Design review of the part built by this model. Coordinates are the model's own, in mm. A direction names the side the tool comes from. Give positions to 0.01 mm unless a question says otherwise; leave off trailing zeros. Write each loop counter-clockwise with the first axis right and the second up, starting at its lowest first coordinate (ties: lowest second). Pieces come first, ordered by that corner, then holes. Notation, with made-up numbers: M 14,66.5 L 23,66.5 A31 ccw 23,93.5 Z; hole C 66.25,74 d9. An arc over 180 degrees is marked long. Answer in a Markdown table with one row per item.
```python
from build123d import *

# Parameters (mm, degrees)
F0_W     = 140
F0_H     = 320
F1_DEPTH = 4.826
F2_W     = 31.75
F2_H     = 31.75
F2_W_2   = 25.4
F2_H_2   = 25.4
F3_DEPTH = 320
F4_W     = 25.4
F4_H     = 25.4
F4_W_2   = 15.874
F4_H_2   = 15.874
F5_DEPTH = 25
F6_R     = 2
F7_DEPTH = 4
F8_R     = 2.5
F8_R_2   = 3
F9_DEPTH = 4


with BuildPart() as f1:
    # F0 (on Top) → F1 (new body)
    with BuildSketch(Plane.XY):
        with Locations((-1.276044, 117.026612)):
            Rectangle(F0_W, F0_H)
    extrude(amount=F1_DEPTH)

    # F2 (on face) → F3 (join)
    with BuildSketch(Plane.XZ.offset(42.973388)):
        with Locations((-55.401044, -15.875)):
            Rectangle(F2_W, F2_H)
        with Locations((-55.401044, -15.875)):
            Rectangle(F2_W_2, F2_H_2, mode=Mode.SUBTRACT)
        with Locations((52.848956, -15.875)):
            Rectangle(F2_W, F2_H)
        with Locations((52.848956, -15.875)):
            Rectangle(F2_W_2, F2_H_2, mode=Mode.SUBTRACT)
    extrude(amount=-F3_DEPTH)

    # F4 (on face) → F5 (join, symmetric)
    with BuildSketch(Plane.XZ.offset(42.973388)):
        with Locations((-55.401044, -15.875)):
            Rectangle(F4_W, F4_H)
        with Locations((-55.401044, -15.875)):
            Rectangle(F4_W_2, F4_H_2, mode=Mode.SUBTRACT)
        with Locations((52.848956, -15.875)):
            Rectangle(F4_W, F4_H)
        with Locations((52.848956, -15.875)):
            Rectangle(F4_W_2, F4_H_2, mode=Mode.SUBTRACT)
    extrude(amount=F5_DEPTH, both=True)

    # F6 (on face) → F7 (cut)
    with BuildSketch(Plane.YZ.offset(-39.526044)):
        with Locations((117.026612, -21.75)):
            Circle(F6_R)
    extrude(amount=-F7_DEPTH, mode=Mode.SUBTRACT)

    # F8 (on face) → F9 (cut)
    with BuildSketch(Plane.XY.offset(4.826)):
        with Locations((-36.276044, -22.973388)):
            Circle(F8_R)
        with Locations((28.723956, -32.973388)):
            Circle(F8_R_2)
    extrude(amount=-F9_DEPTH, mode=Mode.SUBTRACT)


solid = f1.part
```
1) The part is to be moulded in two halves that separate along Z. For faces 6 (the face through (-42.701, 127, -16)), 7 (the face through (40.149, -56, -16)), 8 (the face through (-56, -55, -3.175)), say which applies: released by +Z, released by -Z, zero draft, split by the parting line, or undercut.
Geometry says:
| item | result |
|---|---|
| face 6 | undercut |
| face 7 | zero draft |
| face 8 | released by +Z |
2) Add section A-A (y = 71). Write out the cut boundary in (x, z) (3 decimals).
Geometry says:
| item | result |
|---|---|
| outline | M -71.276,-31.75 L -39.526,-31.75 L -39.526,0 L 36.974,0 L 36.974,-31.75 L 68.724,-31.75 L 68.724,4.826 L -71.276,4.826 Z; hole M -68.101,-28.575 L -42.701,-28.575 L -42.701,-3.175 L -68.101,-3.175 Z; hole M 40.149,-28.575 L 65.549,-28.575 L 65.549,-3.175 L 40.149,-3.175 Z |
3) To check wall thickness, follow probe 1 along X at (y, z) = (146, -15.5); probe 2 along Z at (x, y) = (-65.5, 92) (3 decimals); probe 3 along Z at (x, y) = (-39, 94.5). State the ranges of each line that lie inside material, in increasing order. Write a range as [from, to].
Geometry says:
| item | result |
|---|---|
| probe 1 | [-71.28, -68.1], [-42.7, -39.53], [36.97, 40.15], [65.55, 68.72] |
| probe 2 | [-31.75, -28.575], [-3.175, 4.826] |
| probe 3 | [0, 4.83] |
4) Add section B-B (x = -21). Write out the cut boundary in (y, z).
Geometry says:
| item | result |
|---|---|
| outline | M -42.97,0 L 277.03,0 L 277.03,4.83 L -42.97,4.83 Z |
5) Insertion check: P1, Ø5, axis at x = -33, y = 81, coming from the -Z side; P2, Ø8, axis at x = -58.5, y = -51.5, coming from the +Z side (3 decimals); P3, Ø5, axis at x = -57.5, y = -46, coming from the -Z side (3 decimals). Each pin has a flat end and moves straight along its axis. Give the tip position at first contact, or say it passes through.
Geometry says:
| item | result |
|---|---|
| P1 | z = 0 |
| P2 | z = -3.175 |
| P3 | z = -28.575 |
6) For faces 1 (the face through (36.974, 115, -16)), 2 (the face through (-56, 127, -3.175)), 3 (the face through (53, -56, -3.175)), 4 (the face through (-42.701, -55, -16)), 5 (the face through (60.786, -43, -16)), list the 3-axis set-ups (+Z, -Z, +X, -X, +Y, -Y) from which the entire face can be reached by the end or side of a thin tool; tool diameter is ignored.
Geometry says:
| item | result |
|---|---|
| face 1 | -Z, +Y, -Y |
| face 2 | +Y |
| face 3 | +Z, +X, -X, -Y |
| face 4 | +Z, -Z, -Y |
| face 5 | +Y, -Y |
